from build123d import *

# Parameters (mm, degrees)
BOSS_EXTRUDE1_DEPTH = 15
BOSS_EXTRUDE2_DEPTH = 9
BOSS_EXTRUDE3_DEPTH = 10


with BuildPart() as part:
    # Sketch1 → Boss-Extrude1 (new body)
    with BuildSketch(Plane.XY):
        with BuildLine():
            Line((2, 0), (8, 0))
            ThreePointArc((8, 0), (9.414213562, 0.585786438), (10, 2))
            Line((10, 2), (10, 10))
            ThreePointArc((10, 10), (9.414213562, 11.414213562), (8, 12))
            Line((8, 12), (2, 12))
            ThreePointArc((2, 12), (0.585786438, 11.414213562), (0, 10))
            Line((0, 10), (0, 2))
            ThreePointArc((0, 2), (0.585786438, 0.585786438), (2, 0))
        make_face()
    extrude(amount=BOSS_EXTRUDE1_DEPTH)

    # Sketch2 → Boss-Extrude2 (add)
    with BuildSketch(Plane.XY.offset(15)):
        with BuildLine():
            Line((1, 0), (9, 0))
            ThreePointArc((9, 0), (9.707106781, 0.292893219), (10, 1))
            Line((10, 1), (10, 11))
            ThreePointArc((10, 11), (9.707106781, 11.707106781), (9, 12))
            Line((9, 12), (1, 12))
            ThreePointArc((1, 12), (0.292893219, 11.707106781), (0, 11))
            Line((0, 11), (0, 1))
            ThreePointArc((0, 1), (0.292893219, 0.292893219), (1, 0))
        make_face()
    extrude(amount=BOSS_EXTRUDE2_DEPTH)

    # Sketch3 → Boss-Extrude3 (add)
    with BuildSketch(Plane.XY.offset(24)):
        with BuildLine():
            Line((6.206664687, 6.891044518), (3.793335313, 6.891044518))
            ThreePointArc((3.793335313, 6.891044518), (4.530956841, 4.575219836), (6.5, 6))
            ThreePointArc((6.5, 6), (6.424780164, 6.469043159), (6.206664687, 6.891044518))
        make_face()
    extrude(amount=BOSS_EXTRUDE3_DEPTH)


solid = part.part
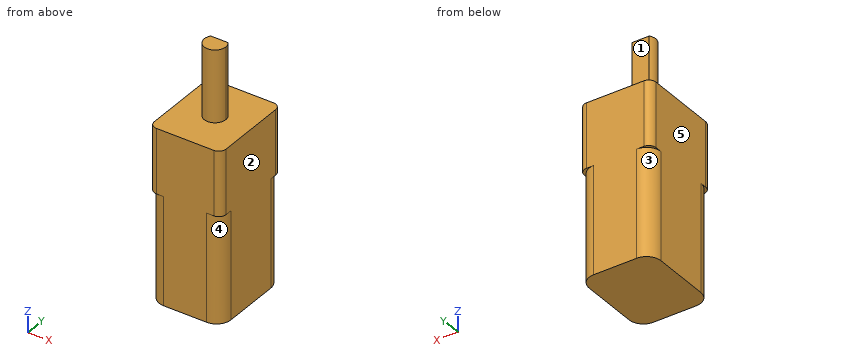
CAD build for the part. Positions are in the model's coordinates, mm. Face numbers are marked on the shaded views. A direction names the side the tool comes from. Round coordinates to 2 decimals unless told otherwise and drop trailing zeros. Order: outer loops, then holes, each group sorted by start corner. A loop starts at its lowest first (then second) coordinate and runs counter-clockwise, first axis right, second up. Notation, with made-up numbers: M 46.5,-38.5 L 69.5,-38.5 A11 ccw 69.5,-19.5 Z; hole C 24,80 d11. An arc over 180 degrees is marked long. Use one line per item in the form item = value.
Q1. Saw through at D-D on x = 7.5. Give the cut face in (y, z).
Recorded:
outline = M 0,0 L 12,0 L 12,24 L 0,24 Z
Q2. Saw through at B-B on x = 5. Give the cut face in (y, z), then the cut area to 3 significant figures.
Recorded:
outline = M 0,0 L 12,0 L 12,24 L 6.89,24 L 6.89,34 L 4.5,34 L 4.5,24 L 0,24 Z
area = 312 mm^2
Q3. Flat gauge pin, fed straight in: P1, Ø0.7, axis at x = 5.5, z = 26.5, coming from the +Y side. Where does the tip first touch, or does it go through?
Recorded:
P1 = 6.89
Q4. Which spindle directions (+Z, -Z, +X, -X, +Y, -Y) get a long thin tool onto all of the face, cutting with end or side? Do the marked faces 1, 2, 3, 4 and 5. Say none if no direction does.
Recorded:
face_1 = +Z, +X, -X, +Y
face_2 = +Z, -Z, +X, +Y, -Y
face_3 = -Z, -X, +Y
face_4 = -Z, +X, -Y
face_5 = +Z, -Z, -X, +Y, -Y
Q5. Probe L1, parallel to Z at x = 5, y = 10.5; L2, parallel to Y at x = 8.5, z = 6; L3, parallel to X at y = 11.5, z = 17. List the from-to ranges inside material, lowest first.
Recorded:
L1 = 0 to 24
L2 = 0.06 to 11.94
L3 = 0.13 to 9.87
Q6. Saw through at A-A on z = 14.5. Give the cut face in (x, y).
Recorded:
outline = M 0,2 A2 ccw 2,0 L 8,0 A2 ccw 10,2 L 10,10 A2 ccw 8,12 L 2,12 A2 ccw 0,10 Z
Q7. Saw through at C-C on y = 3.75. Give the cut face in (x, z), then the cut area to 3 significant figures.
Recorded:
outline = M 0,0 L 10,0 L 10,24 L 0,24 Z
area = 240 mm^2
